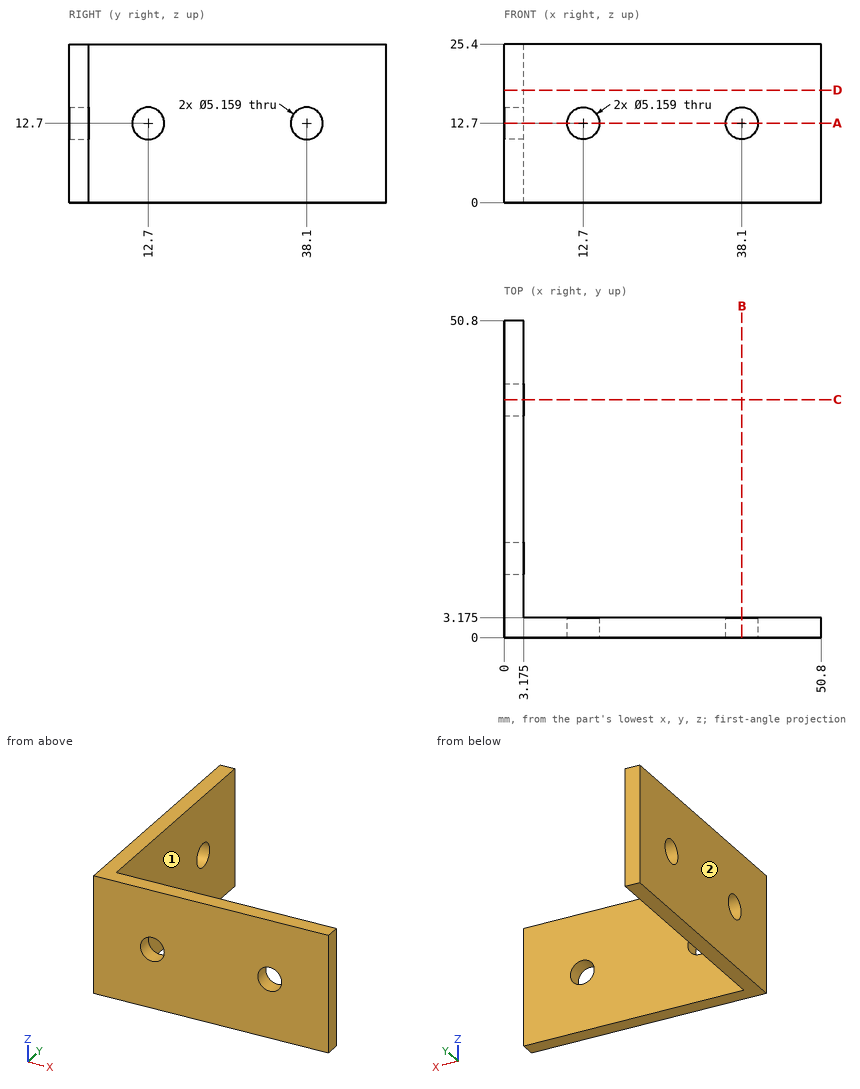
Answer from the drawing. Dimensions are ordinates in mm from the lowest x, y and z of the part. A direction names the side the tool comes from. Coordinates: 2 decimals unless noted, no trailing zeros. Order: outer loops, then holes, each group sorted by start corner. A loop starts at its lowest first (then second) coordinate and runs counter-clockwise, first axis right, second up. Notation, with made-up numbers: (-14.5, 28.25) - (9.5, 28.25) arc R24 cw to (9.5, 57.25) - close; hole circle Ø7 at (43, 8). An arc over 180 degrees is marked (long way). Put each result on its own line as item: value. Start each with the question number.
1) For the marked faces 1 and 2, determine the directions among +Z, -Z, +X, -X, +Y, -Y from which every point of the face is accessible in a straight line to the end or side of a thin tool.
2) Find section D-D (z = 18). Give the vertices of the cut face in (x, y) (1 decimal).
3) Find section A-A (z = 12.7). Give the vertices of the cut face in (x, y) (1 decimal), plus the area to 3 significant figures.
4) Flat-ended cylindrical pins translate along their axes: pin 1 (4 mm diameter, centred on x = 31.5, z = 14.5, fed in from +Y) (3 decimals); pin 2 (1.5 mm diameter, centred on y = 5.5, z = 15.5, fed in from +X) (3 decimals). Find the tip coordinate at first contact, or state that the pin passes through.
5) Find section B-B (x = 38.1). Give the vertices of the cut face in (y, z) (1 decimal).
6) Find the intervals of material crossed by line 1 (X direction, y = 1.15, z = 12.7); line 2 (X direction, y = 42.5, z = 24) (1 decimal), in increasing order. Write a range as from..to.
Results list:
1. face 1: +Z, -Z, +X, +Y
1. face 2: +Z, -Z, -X, +Y, -Y
2. outline: (0, 0) - (50.8, 0) - (50.8, 3.2) - (3.2, 3.2) - (3.2, 50.8) - (0, 50.8) - close
3. outline: (0, 0) - (10.1, 0) - (10.1, 3.2) - (3.2, 3.2) - (3.2, 10.1) - (0, 10.1) - close; (0, 15.3) - (3.2, 15.3) - (3.2, 35.5) - (0, 35.5) - close; (0, 40.7) - (3.2, 40.7) - (3.2, 50.8) - (0, 50.8) - close; (15.3, 0) - (35.5, 0) - (35.5, 3.2) - (15.3, 3.2) - close; (40.7, 0) - (50.8, 0) - (50.8, 3.2) - (40.7, 3.2) - close
3. area: 247 mm^2
4. pin 1: stops at y = 3.175
4. pin 2: stops at x = 3.175
5. outline: (0, 0) - (3.2, 0) - (3.2, 10.1) - (0, 10.1) - close; (0, 15.3) - (3.2, 15.3) - (3.2, 25.4) - (0, 25.4) - close
6. line 1: x = 0..10.12, 15.28..35.52, 40.68..50.8
6. line 2: x = 0..3.2
